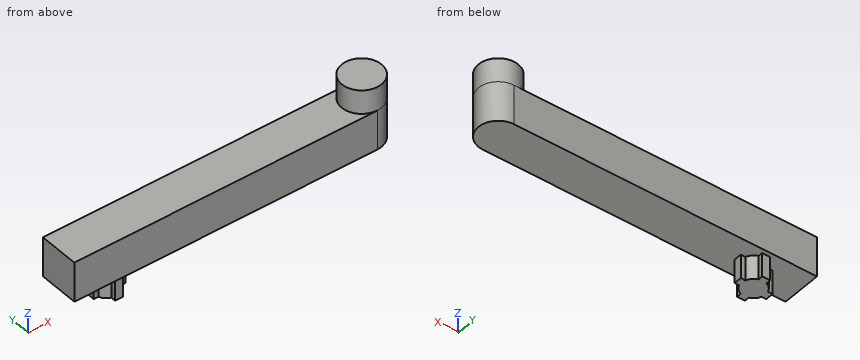
```python
from build123d import *

# Parameters (mm, degrees)
F0_R     = 2.5
F1_DEPTH = 3
F3_DEPTH = 5
F5_DEPTH = 3


with BuildPart() as f1:
    # F0 (on Top) → F1 (new body)
    with BuildSketch(Plane.XY):
        Circle(F0_R)
    extrude(amount=-F1_DEPTH)

    # F2 (on face) → F3 (join)
    with BuildSketch(Plane(origin=(0, 0, -3), x_dir=(1, 0, 0), z_dir=(0, 0, -1))):
        with BuildLine():
            Line((-38.1, -2.5), (0, -2.5))
            ThreePointArc((0, -2.5), (2.5, 0), (0, 2.5))
            Line((0, 2.5), (-38.1, 2.5))
            Line((-38.1, 2.5), (-38.1, -2.5))
        make_face()
    extrude(amount=F3_DEPTH)

    # F4 (on face) → F5 (join)
    with BuildSketch(Plane(origin=(0, 0, -8), x_dir=(1, 0, 0), z_dir=(0, 0, -1))):
        with BuildLine():
            Line((-32.6, 2), (-32.6, 1.414214))
            ThreePointArc((-32.6, 1.414214), (-33.16066, 1.06066), (-33.514214, 0.5))
            Line((-33.514214, 0.5), (-34.1, 0.5))
            Line((-34.1, 0.5), (-34.1, -0.5))
            Line((-34.1, -0.5), (-33.514214, -0.5))
            ThreePointArc((-33.514214, -0.5), (-33.16066, -1.06066), (-32.6, -1.414214))
            Line((-32.6, -1.414214), (-32.6, -2))
            Line((-32.6, -2), (-31.6, -2))
            Line((-31.6, -2), (-31.6, -1.414214))
            ThreePointArc((-31.6, -1.414214), (-31.03934, -1.06066), (-30.685786, -0.5))
            Line((-30.685786, -0.5), (-30.1, -0.5))
            Line((-30.1, -0.5), (-30.1, 0.5))
            Line((-30.1, 0.5), (-30.685786, 0.5))
            ThreePointArc((-30.685786, 0.5), (-31.03934, 1.06066), (-31.6, 1.414214))
            Line((-31.6, 1.414214), (-31.6, 2))
            Line((-31.6, 2), (-32.6, 2))
        make_face()
    extrude(amount=F5_DEPTH)


solid = f1.part
```
Geometry check sheet. Reference: the model listing, model coordinates, mm. Coordinates: 2 decimals unless noted, no trailing zeros. Order: outer loops, then holes, each group sorted by start corner. A loop starts at its lowest first (then second) coordinate and runs counter-clockwise, first axis right, second up.
Q1. Sectioned sample at C-C on y = 0. Record the cut outline in (x, z).
Reply:
outline: (-38.1, -8) - (-34.1, -8) - (-34.1, -11) - (-30.1, -11) - (-30.1, -8) - (2.5, -8) - (2.5, 0) - (-2.5, 0) - (-2.5, -3) - (-38.1, -3) - close
Q2. Depth check by flat-ended pin: pin 1 Ø6 at (x, z) = (-29.5, -10) entering from -Y; pin 2 Ø1.1 at (x, z) = (-32, -9) entering from +Y; pin 3 Ø1.5 at (x, y) = (-11.5, -0.5) entering from -Z; pin 4 Ø0.8 at (y, z) = (0, -9.5) entering from -X. Enter the tip coordinate at first touch or a pass-through.
Reply:
pin 1: stops at y = -2.5
pin 2: stops at y = 2
pin 3: stops at z = -8
pin 4: stops at x = -34.1
Q3. Sectioned sample at D-D on x = -26.5. Record the cut outline in (y, z).
Reply:
outline: (-2.5, -8) - (2.5, -8) - (2.5, -3) - (-2.5, -3) - close
Q4. Thickness scan on probe 1 along Z at (x, y) = (-24.5, 2.05); probe 2 along X at (y, z) = (0.7, -0.5); probe 3 along X at (y, z) = (1.5, -1). Record the ranges inside material, lowest first.
Reply:
probe 1: z = -8 to -3
probe 2: x = -2.4 to 2.4
probe 3: x = -2 to 2
Q5. Sectioned sample at A-A on z = -9.5. Record the cut outline in (x, y).
Reply:
outline: (-34.1, -0.5) - (-33.51, -0.5) arc R1.5 ccw to (-32.6, -1.41) - (-32.6, -2) - (-31.6, -2) - (-31.6, -1.41) arc R1.5 ccw to (-30.69, -0.5) - (-30.1, -0.5) - (-30.1, 0.5) - (-30.69, 0.5) arc R1.5 ccw to (-31.6, 1.41) - (-31.6, 2) - (-32.6, 2) - (-32.6, 1.41) arc R1.5 ccw to (-33.51, 0.5) - (-34.1, 0.5) - close
Q6. Sectioned sample at B-B on x = -2. Record the cut outline in (y, z), and give its area (3 significant figures).
Reply:
outline: (-2.5, -8) - (2.5, -8) - (2.5, -3) - (1.5, -3) - (1.5, 0) - (-1.5, 0) - (-1.5, -3) - (-2.5, -3) - close
area: 34.0 mm2
